```python
from build123d import *

# Parameters (mm, degrees)
SKETCH1_R           = 20.5
SKETCH1_R_2         = 5.25
BOSS_EXTRUDE1_DEPTH = 10
SKETCH2_R           = 8
CUT_EXTRUDE1_DEPTH  = 5
SKETCH5_R           = 1.5
CUT_EXTRUDE2_DEPTH  = 10


with BuildPart() as part:
    # Sketch1 → Boss-Extrude1 (new body)
    with BuildSketch(Plane(origin=(0, 0, 0), x_dir=(1, 0, 0), z_dir=(0, 1, 0))):
        with Locations(Location((0, 0, 0), (0, 0, 270))):
            Circle(SKETCH1_R)
        with Locations(Location((0, 0, 0), (0, 0, 270))):
            Circle(SKETCH1_R_2, mode=Mode.SUBTRACT)
    extrude(amount=BOSS_EXTRUDE1_DEPTH)

    # Sketch2 → Cut-Extrude1 (cut)
    with BuildSketch(Plane(origin=(0, 10, 0), x_dir=(1, 0, 0), z_dir=(0, 1, 0))):
        with Locations(Location((0, 0, 0), (0, 0, 270))):
            Circle(SKETCH2_R)
    extrude(amount=-CUT_EXTRUDE1_DEPTH, mode=Mode.SUBTRACT)

    # Sketch5 → Cut-Extrude2 (cut)
    with BuildSketch(Plane(origin=(0, 10, 0), x_dir=(1, 0, 0), z_dir=(0, 1, 0))):
        with Locations(Location((0, 15.5, 0), (0, 0, 270))):
            Circle(SKETCH5_R)
        with Locations(Location((15.5, 0, 0), (0, 0, 270))):
            Circle(SKETCH5_R)
        with Locations(Location((0, -15.5, 0), (0, 0, 270))):
            Circle(SKETCH5_R)
        with Locations(Location((-15.5, 0, 0), (0, 0, 270))):
            Circle(SKETCH5_R)
    extrude(amount=-CUT_EXTRUDE2_DEPTH, mode=Mode.SUBTRACT)


solid = part.part
```
Input: part model. Units: mm. Frame: model coordinates. A direction names the side the tool comes from. Give positions to 0.01 mm unless a question says otherwise; leave off trailing zeros. Order: outer loops, then holes, each group sorted by start corner. A loop starts at its lowest first (then second) coordinate and runs counter-clockwise, first axis right, second up.
1. Section B-B on z = -3. Return the cut outline in (x, y).
Derived:
outline: (-20.28, 0) - (-4.31, 0) - (-4.31, 5) - (-7.42, 5) - (-7.42, 10) - (-20.28, 10) - close; (4.31, 0) - (20.28, 0) - (20.28, 10) - (7.42, 10) - (7.42, 5) - (4.31, 5) - close
2. Section A-A on x = 0. Return the cut outline in (y, z), and give its area (4 significant figures).
Derived:
outline: (0, -20.5) - (10, -20.5) - (10, -17) - (0, -17) - close; (0, -14) - (10, -14) - (10, -8) - (5, -8) - (5, -5.25) - (0, -5.25) - close; (0, 5.25) - (5, 5.25) - (5, 8) - (10, 8) - (10, 14) - (0, 14) - close; (0, 17) - (10, 17) - (10, 20.5) - (0, 20.5) - close
area: 217.5 mm2
3. Reachability of faces 4 (the cylindrical face through (-7.81, 7.54, -1.73)), 5 (the cylindrical face through (-15.05, 5.07, 1.43)) from +Z, -Z, +X, -X, +Y, -Y: full face, straight path, thin tool, end or side. Return the list, or none.
Derived:
face 4: +Y
face 5: +Y, -Y
4. Material intervals for L1, parallel to X at y = 1.15, z = 0; L2, parallel to X at y = 7.5, z = 0; L3, parallel to X at y = 7.5, z = 15.5, sorted ascending.
Derived:
L1: x = -20.5 to -17, -14 to -5.25, 5.25 to 14, 17 to 20.5
L2: x = -20.5 to -17, -14 to -8, 8 to 14, 17 to 20.5
L3: x = -13.42 to -1.5, 1.5 to 13.42
5. Section C-C on y = 2. Return the cut outline in (x, z).
Derived:
outline: circle Ø41 at (0, 0); hole circle Ø3 at (-15.5, 0); hole circle Ø10.5 at (0, 0); hole circle Ø3 at (0, -15.5); hole circle Ø3 at (0, 15.5); hole circle Ø3 at (15.5, 0)
6. Mould query, pull axis X, two halves, no side actions, for faces 1 (the flat face through (-4, 0, 4)), 2 (the cylindrical face through (-20.013, 4.93, -4.444)), 3 (the cylindrical face through (0, 5, -17)). Classes: released by +X, released by -X, zero draft, split by the parting line, or undercut.
Derived:
face 1: zero draft
face 2: split by the parting line
face 3: undercut
7. Pin query (flat end, axial travel): pin 1 (4 mm diameter, centred on y = 4.5, z = 6, fed in from -X); pin 2 (13.5 mm diameter, centred on x = 0, z = 0, fed in from +Y); pin 3 (1.5 mm diameter, centred on x = 12, y = 5, fed in from +Z). Return the tip coordinate at first contact, or that it passes through.
Derived:
pin 1: stops at x = -20.11
pin 2: stops at y = 5
pin 3: stops at z = 17.14
8. Section D-D on x = -16. Return the cut outline in (y, z), and give its area (3 significant figures).
Derived:
outline: (0, -12.82) - (10, -12.82) - (10, -1.41) - (0, -1.41) - close; (0, 1.41) - (10, 1.41) - (10, 12.82) - (0, 12.82) - close
area: 228 mm2
